Here's the drawing with two shaded views (mm, measured from the low corner). I have some questions. A direction names the side the tool comes from. Give positions to 0.01 mm unless a question says otherwise; leave off trailing zeros. Write each loop counter-clockwise with the first axis right and the second up, starting at its lowest first coordinate (ties: lowest second). Pieces come first, ordered by that corner, then holes. Notation, with made-up numbers: (-4.5, 39.25) - (20.5, 39.25) arc R16 cw to (20.5, 63.25) - close; hole circle Ø6 at (86, 9). An arc over 180 degrees is marked (long way). Use one line per item in the form item = value.
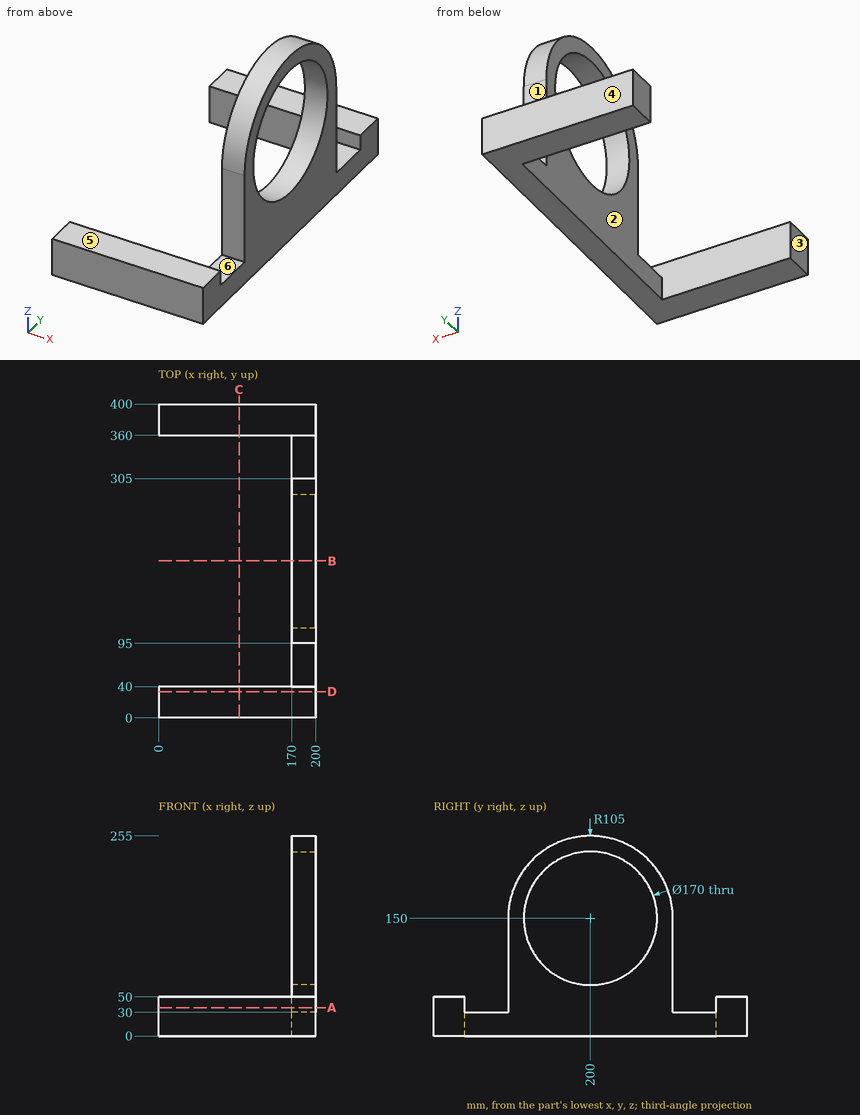
1. Imagine slicing it at D-D, the plane y = 33.5. List the corners of the cut face in (x, z) for me.
Response values:
outline = (0, 0) - (200, 0) - (200, 50) - (0, 50) - close
2. If we mould it in two halves opening along Y, with no side actions, what happens to the marked faces 4, 5 and 6? For each: pulls with the +Y half, pulls with the -Y half, needs draft (parallel to the pull), parting line crosses it, or undercut.
Response values:
face_4 = pulls with the +Y half
face_5 = needs draft
face_6 = undercut
3. If I drill on line 1 (Y direction, x = 194, z = 150); line 2 (Y direction, x = 85.5, z = 49); line 3 (X direction, y = 333, z = 11.5), over which ranges is the centre line in solid material (lowest first)? Write a range as from..to.
Response values:
line_1 = 95..115, 285..305
line_2 = 0..40, 360..400
line_3 = 170..200
4. Which directions (+Z, -Z, +X, -X, +Y, -Y) give clear straight access to the entire face, cutting with the end or side of a thin tool? Please do the marked faces 1, 2 and 3.
Response values:
face_1 = +Z, +X, -X
face_2 = +Z, -Z, -X
face_3 = +Z, -Z, -X, +Y, -Y
5. Imagine slicing it at A-A, the plane z = 36. List the corners of the cut face in (x, y) for me.
Response values:
outline = (0, 0) - (200, 0) - (200, 40) - (0, 40) - close; (0, 360) - (200, 360) - (200, 400) - (0, 400) - close; (170, 95) - (200, 95) - (200, 305) - (170, 305) - close
6. Imagine slicing it at C-C, the plane x = 102.5. List the corners of the cut face in (y, z) for me, and give its area (3 significant figures).
Response values:
outline = (0, 0) - (40, 0) - (40, 50) - (0, 50) - close; (360, 0) - (400, 0) - (400, 50) - (360, 50) - close
area = 4,000 mm²
7. Imagine slicing it at B-B, the plane y = 200. List the corners of the cut face in (x, z) for me, and give its area (3 significant figures).
Response values:
outline = (170, 0) - (200, 0) - (200, 65) - (170, 65) - close; (170, 235) - (200, 235) - (200, 255) - (170, 255) - close
area = 2,550 mm²
8. For pin 1 (9 mm diameter, centred on x = 188, z = 71.5, fed in from +Y); pin 2 (1.5 mm diameter, centred on y = 305.5, z = 67, fed in from -X); pin 3 (15 mm diameter, centred on x = 190.5, z = 120, fed in from -Y), each with a flat end and sliding along its axis, tell me the tip position at first contact or that it passes through.
Response values:
pin_1 = 305
pin_2 = 170
pin_3 = 95
